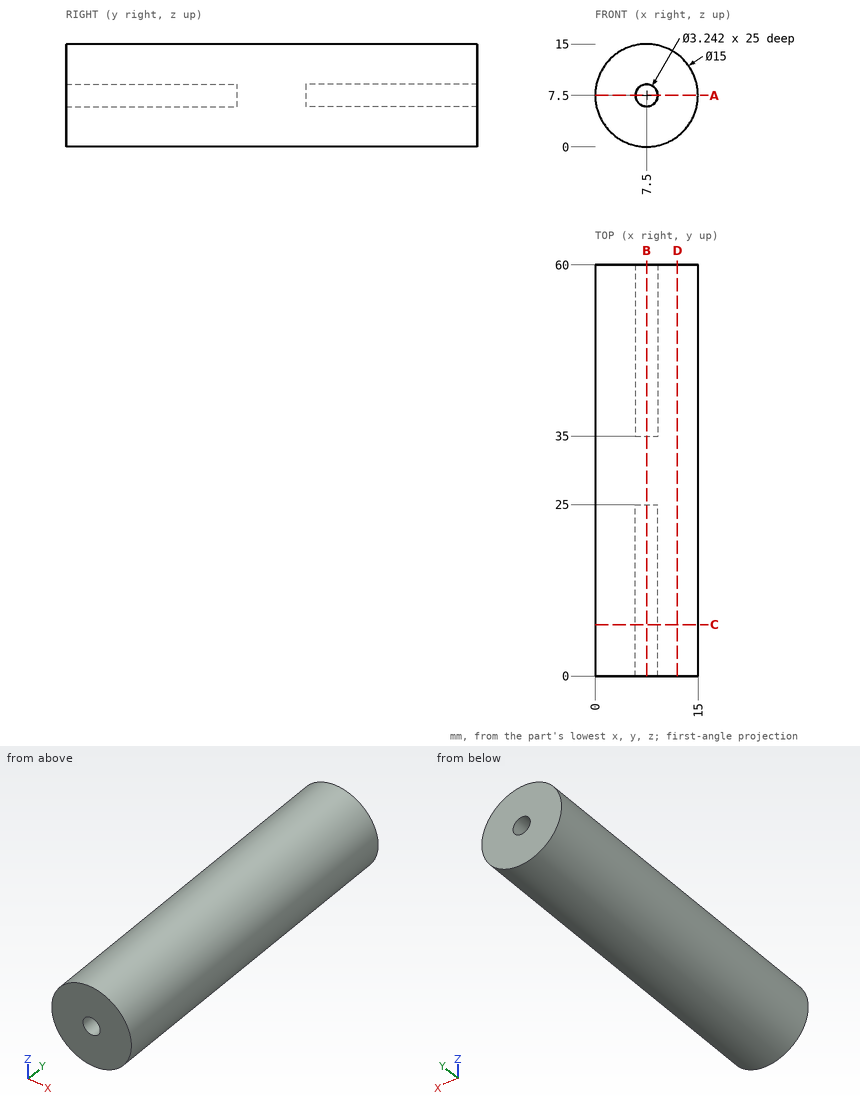
Verification items for this drawing (mm, ordinates from the low corner). Give positions to 0.01 mm unless a question says otherwise; leave off trailing zeros. Loops run counter-clockwise (first coordinate to the right, second up) from the corner with the lowest first, then second, coordinate; pieces in that order, holes last. Notation, with made-up numbers: M -2,5 L 56,5 A27 cw 56,24 Z; hole C -19.5,-12.5 d2. An arc over 180 degrees is marked long. Answer as a JSON object with one key per item and string values. Group by question number.
Q1. Cross-section at A-A on z = 7.5. Record the cut outline in (x, y).
Q2. Cross-section at C-C on y = 7.5. Record the cut outline in (x, z), then the cut area to 3 significant figures.
Q3. Material ranges on line 1 along Z through (x, y) = (7.5, 5.5); line 2 along Y through (x, z) = (7.5, 6.25); line 3 along Z through (x, y) = (8, 22), recorded low to high. Write a range as [from, to].
Q4. Cross-section at B-B on x = 7.5. Record the cut outline in (y, z).
Q5. Go/stop test with flat-tipped pins: P1, Ø5, axis at y = 19.5, z = 3, coming from the +X side; P2, Ø1, axis at y = 15, z = 5.5, coming from the -X side; P3, Ø1, axis at x = 10.5, y = 32, coming from the -Z side. Record where each tip stops, or that it passes through.
Q6. Cross-section at D-D on x = 12. Record the cut outline in (y, z).
Evaluation:
{
 "1": {"outline": "M 0,0 L 5.88,0 L 5.88,25 L 9.12,25 L 9.12,0 L 15,0 L 15,60 L 9.12,60 L 9.12,35 L 5.88,35 L 5.88,60 L 0,60 Z"},
 "2": {"outline": "C 7.5,7.5 d15; hole C 7.5,7.5 d3.24", "area": "168 mm2"},
 "3": {"line 1": "z = [0, 5.88], [9.12, 15]", "line 2": "y = [25, 35]", "line 3": "z = [0.02, 5.96], [9.04, 14.98]"},
 "4": {"outline": "M 0,0 L 60,0 L 60,5.88 L 35,5.88 L 35,9.12 L 60,9.12 L 60,15 L 0,15 L 0,9.12 L 25,9.12 L 25,5.88 L 0,5.88 Z"},
 "5": {"P1": "stops at x = 14.73", "P2": "stops at x = 0.15", "P3": "stops at z = 0.43"},
 "6": {"outline": "M 0,1.5 L 60,1.5 L 60,13.5 L 0,13.5 Z"}
}
